Could you check a few things on this drawing? It's one solid part, dimensions in mm from its lowest x, y, z. Round coordinates to 2 decimals unless told otherwise and drop trailing zeros. Order: outer loops, then holes, each group sorted by start corner. A loop starts at its lowest first (then second) coordinate and runs counter-clockwise, first axis right, second up. Notation, with made-up numbers: (50.5, 42) - (101.5, 42) arc R27 ccw to (101.5, 73) - close; hole circle Ø8 at (27.5, 10). An arc over 180 degrees is marked (long way). Use one line per item in the form item = value.
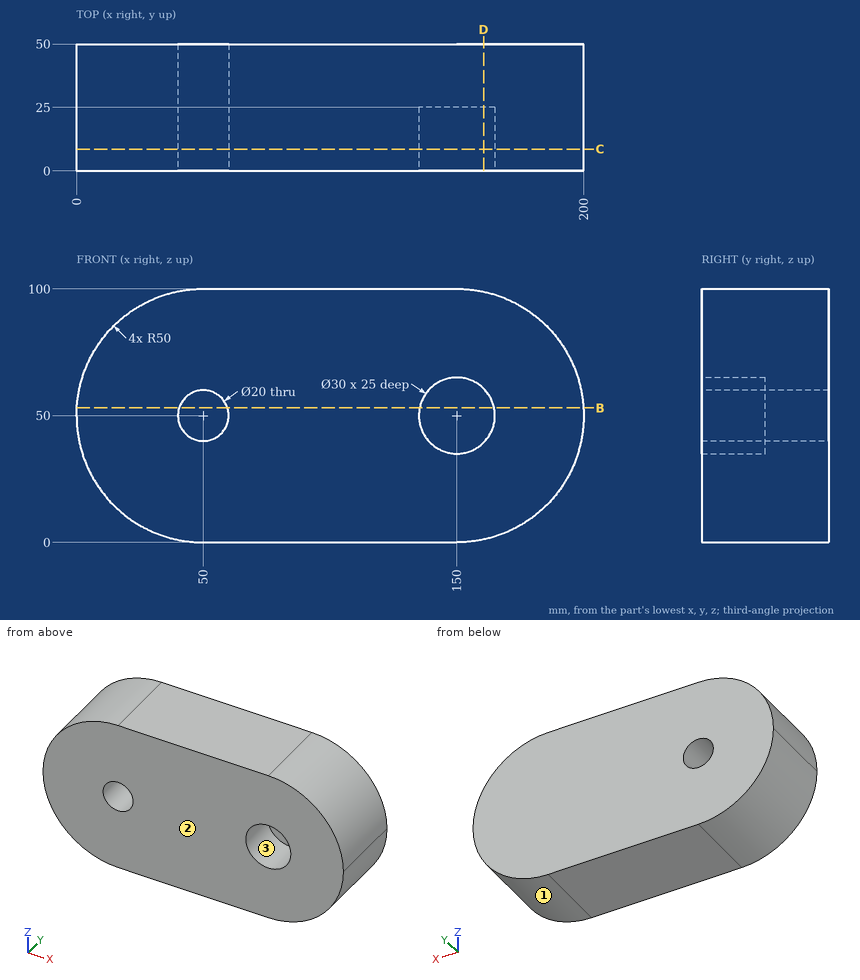
Item 1: If we mould it in two halves opening along X, with no side actions, what happens to the marked faces 1, 2 and 3? For each: released by +X, released by -X, zero draft, split by the parting line, or undercut.
Found:
face_1 = released by +X
face_2 = zero draft
face_3 = undercut
Item 2: Will these pins go through, and if not, where does the flat tip stop? P1, Ø8, axis at y = 32, z = 57.5, coming from the -X side; P2, Ø16, axis at x = 50, z = 50, coming from the -Y side; P3, Ø2, axis at x = 43, y = 28.5, coming from the +Z side; P4, Ø24, axis at x = 150, z = 50, coming from the -Y side.
Found:
P1 = 0.12
P2 = through
P3 = 99.64
P4 = 25
Item 3: I need wall thicknesses on L1, parallel to X at y = 14.75, z = 50; L2, parallel to X at y = 47.5, z = 49.5; L3, parallel to X at y = 12.5, z = 58. Which ranges of each line are inside material? Lowest first, please.
Found:
L1 = 0 to 40, 60 to 135, 165 to 200
L2 = 0 to 40.01, 59.99 to 200
L3 = 0.64 to 44, 56 to 137.31, 162.69 to 199.36
Item 4: Imagine slicing it at D-D on x = 160.5. Please give me the cut outline in (y, z) (3 decimals), plus the area to 3 significant figures.
Found:
outline = (0, 1.115) - (50, 1.115) - (50, 98.885) - (0, 98.885) - (0, 60.712) - (25, 60.712) - (25, 39.288) - (0, 39.288) - close
area = 4,350 mm2
Item 5: Imagine slicing it at C-C on y = 8.5. State how many separate pieces and enclosed holes the cut face has, plus the area to 3 significant figures.
Found:
separate_pieces = 1
enclosed_holes = 2
area = 16,800 mm2
Item 6: Imagine slicing it at B-B on z = 53. Please give me the cut outline in (x, y), plus the area to 3 significant figures.
Found:
outline = (0.09, 0) - (40.46, 0) - (40.46, 50) - (0.09, 50) - close; (59.54, 0) - (135.3, 0) - (135.3, 25) - (164.7, 25) - (164.7, 0) - (199.91, 0) - (199.91, 50) - (59.54, 50) - close
area = 8,300 mm2
